```python
from build123d import *

# Parameters (mm, degrees)
F0_W     = 68
F0_H     = 32
F0_W_2   = 66.0000007396
F0_H_2   = 30
F2_DEPTH = 1.5
F5_START = 0.9
F3_W     = 9.7086578608
F3_H     = 13.6771607213
F5_DEPTH = 2.3
F6_START = 1
F1_W     = 13.5039854795
F1_H     = 7.9890675843
F1_W_2   = 10.1785697043
F1_W_3   = 10.0000035018
F1_H_2   = 7.8571438789
F6_DEPTH = 4.6
F7_START = 1.5
F4_W     = 54.7266360372
F4_H     = 8.1930877641
F7_DEPTH = 4


with BuildPart() as f2:
    # F0 (on Top) → F2 (new body)
    with BuildSketch(Plane.XY):
        with Locations((0, -0.0852976367)):
            Rectangle(F0_W, F0_H)
        with Locations((0, -0.0852976367)):
            Rectangle(F0_W_2, F0_H_2, mode=Mode.SUBTRACT)
    extrude(amount=F2_DEPTH)

    # F3 (on Top) → F5 (cut)
    with BuildSketch(Plane.XY.offset(F5_START)):
        with Locations((-30.4173231125, 1.8361529801)):
            Rectangle(F3_W, F3_H)
    extrude(amount=F5_DEPTH, mode=Mode.SUBTRACT)

    # F1 (on Top) → F6 (cut)
    with BuildSketch(Plane.XY.offset(F6_START)):
        with Locations((-19.5872941986, -13.5481059551)):
            Rectangle(F1_W, F1_H)
        with Locations((8.9285718277, -13.5481059551)):
            Rectangle(F1_W_2, F1_H)
        with Locations((21.8750005588, -13.4821441025)):
            Rectangle(F1_W_3, F1_H_2)
    extrude(amount=F6_DEPTH, mode=Mode.SUBTRACT)

    # F4 (on Top) → F7 (cut)
    with BuildSketch(Plane.XY.offset(F7_START)):
        with Locations((0.0114953145, 13.3686042391)):
            Rectangle(F4_W, F4_H)
    extrude(amount=F7_DEPTH, mode=Mode.SUBTRACT)


solid = f2.part
```
Design review of the part built by this model. Coordinates are the model's own, in mm. A direction names the side the tool comes from. Coordinates: 2 decimals unless noted, no trailing zeros. Order: outer loops, then holes, each group sorted by start corner. A loop starts at its lowest first (then second) coordinate and runs counter-clockwise, first axis right, second up.
1) Take a section at B-B, the plane x = -2.5. Give the boundary of the cut face in (y, z).
2) Wall thickness on line 1 along X through (y, z) = (-14, 0.35); line 2 along Y through (x, z) = (-22, 0.35); line 3 along Y through (x, z) = (9, 1.45): over which ranges is each line inside the solid? List them lowest first.
3) For faces 5 (the flat face through (-33, -0.3, 0.6)), 6 (the flat face through (2.4, 15.4, 1.5)), list the 3-axis set-ups (+Z, -Z, +X, -X, +Y, -Y) from which the entire face can be reached by the end or side of a thin tool; tool diameter is ignored.
4) Clearance check with flat-ended pins moving along their axes: pin 1 (1.1 mm diameter, centred on x = -33.5, y = 2.5, fed in from +Z); pin 2 (0.5 mm diameter, centred on x = 9, y = -15.5, fed in from +Z). State where each tip first meets the part, or that it passes through.
5) Take a section at A-A, the plane y = 7.5. Give the boundary of the cut face in (x, z).
6) Mouldability with a two-part tool opening along X and no side actions: class faces 1 (the flat face through (0, 14.915, 1)), 2 (the flat face through (-34, -0.3, 0.6)), 3 (the flat face through (0, -15.085, 1)), 4 (the flat face through (-0.2, 15.4, 0)) as +X half, -X half, draft (parallel to the pull), parting line (faces both ways), or undercut.
Returned:
1. outline: (-16.09, 0) - (-15.09, 0) - (-15.09, 1.5) - (-16.09, 1.5) - close; (14.91, 0) - (15.91, 0) - (15.91, 1.5) - (14.91, 1.5) - close
2. line 1: x = -34 to -33, 33 to 34
2. line 2: y = -16.09 to -15.09, 14.91 to 15.91
2. line 3: y = 14.91 to 15.91
3. face 5: +Z, -Z
3. face 6: +Z, +X, -X, +Y, -Y
4. pin 1: stops at z = 0.9
4. pin 2: stops at z = 1
5. outline: (-34, 0) - (-33, 0) - (-33, 0.9) - (-34, 0.9) - close; (33, 0) - (34, 0) - (34, 1.5) - (33, 1.5) - close
6. face 1: undercut
6. face 2: -X half
6. face 3: undercut
6. face 4: draft
